from build123d import *

# Parameters (mm, degrees)
BOSS_EXTRUDE1_DEPTH     = 10
CUT_EXTRUDE1_DEPTH      = 333.565782966
CUT_EXTRUDE1_DEPTH_BACK = 333.565782966
SKETCH2_R               = 1.6
FILLET2_R               = 5
CUT_EXTRUDE3_DEPTH      = 333.565782966
CUT_EXTRUDE3_DEPTH_BACK = 333.565782966
SKETCH4_R               = 1.6
FILLET3_R               = 10


with BuildPart() as part:
    # Sketch1 → Boss-Extrude1 (new body)
    with BuildSketch(Plane(origin=(0, 0, 0), x_dir=(1, 0, 0), z_dir=(0, 1, 0))):
        Polygon((0, 120), (0, 151.005050634), (70, 320), (90, 320), (90, 170), (40, 120), (40, 0), (0, 0), align=None)
        Polygon((20, 147.026803286), (70, 267.737481405), (70, 178.284271247), (31.715728753, 140), (20, 140), align=None, mode=Mode.SUBTRACT)
    extrude(amount=BOSS_EXTRUDE1_DEPTH)

    # Sketch2 → Cut-Extrude1 (cut, two sides: drawn at the far end of the back side and taken through both)
    with BuildSketch(Plane(origin=(0, 10, 0), x_dir=(1, 0, 0), z_dir=(0, 1, 0)).offset(-CUT_EXTRUDE1_DEPTH_BACK)):
        with Locations(Location((10, 110, 0), (0, 0, 270))):
            Circle(SKETCH2_R)
        with Locations(Location((30, 110, 0), (0, 0, 270))):
            Circle(SKETCH2_R)
        with Locations(Location((10, 10, 0), (0, 0, 270))):
            Circle(SKETCH2_R)
        with Locations(Location((30, 10, 0), (0, 0, 270))):
            Circle(SKETCH2_R)
    extrude(amount=CUT_EXTRUDE1_DEPTH + CUT_EXTRUDE1_DEPTH_BACK, mode=Mode.SUBTRACT)

    # Fillet2
    fillet2_edges = [part.edges().sort_by_distance(p)[0] for p in [
        (20, 5, -147.026803286),
        (20, 5, -140),
        (31.715728753, 5, -140),
        (70, 5, -178.284271247),
        (70, 5, -267.737481405),
    ]]
    fillet(fillet2_edges, radius=FILLET2_R)

    # Sketch4 → Cut-Extrude3 (cut, two sides: drawn at the far end of the back side and taken through both)
    with BuildSketch(Plane(origin=(0, 10, 0), x_dir=(1, 0, 0), z_dir=(0, 1, 0)).offset(-CUT_EXTRUDE3_DEPTH_BACK)):
        with Locations(Location((85, 310, 0), (0, 0, 270))):
            Circle(SKETCH4_R)
        with Locations(Location((85, 245, 0), (0, 0, 270))):
            Circle(SKETCH4_R)
        with Locations(Location((85, 180, 0), (0, 0, 270))):
            Circle(SKETCH4_R)
    extrude(amount=CUT_EXTRUDE3_DEPTH + CUT_EXTRUDE3_DEPTH_BACK, mode=Mode.SUBTRACT)

    # Fillet3
    fillet3_edges = [part.edges().sort_by_distance(p)[0] for p in [
        (0, 5, -151.005050634),
        (70, 5, -320),
        (90, 5, -320),
        (90, 5, -170),
        (40, 5, -120),
        (40, 5, 0),
        (0, 5, 0),
    ]]
    fillet(fillet3_edges, radius=FILLET3_R)


solid = part.part
CAD build for the part. Positions are in the model's coordinates, mm. A direction names the side the tool comes from. Give positions to 0.01 mm unless a question says otherwise; leave off trailing zeros. Loops run counter-clockwise (first coordinate to the right, second up) from the corner with the lowest first, then second, coordinate; pieces in that order, holes last. Notation, with made-up numbers: M 72.5,59.25 L 119.5,59.25 A21 ccw 119.5,68.25 Z; hole C 78.25,20.5 d5. An arc over 180 degrees is marked long. Write each question's results on one line, items separated by ' | '.
Q1. Band-saw the part on A-A on y = 8. Give the number of separate pieces and of enclosed holes in the cut face, and give its area (3 significant figures).
Geometry check:
separate pieces: 1 | enclosed holes: 8 | area: 13,000 mm²
Q2. Band-saw the part on B-B on x = 52.5. Write the cut outline in (y, z), and give its area (3 significant figures).
Geometry check:
outline: M 0,-277.75 L 10,-277.75 L 10,-225.49 L 0,-225.49 Z; M 0,-160.78 L 10,-160.78 L 10,-132.5 L 0,-132.5 Z | area: 805 mm²
Q3. Probe probe 1 along X at (y, z) = (7.75, -110); probe 2 along Z at (x, y) = (85, 6); probe 3 along X at (y, z) = (4, -180). List the from-to ranges inside material, lowest first.
Geometry check:
probe 1: x = 0 to 8.4, 11.6 to 28.4, 31.6 to 40 | probe 2: z = -318.66 to -311.6, -308.4 to -246.6, -243.4 to -181.6, -178.4 to -165 | probe 3: x = 12.01 to 33.66, 69.99 to 83.4, 86.6 to 90
Q4. Band-saw the part on C-C on z = -156. Write the cut outline in (x, y), and give its area (3 significant figures).
Geometry check:
outline: M 2.07,0 L 23.72,0 L 23.72,10 L 2.07,10 Z; M 47.72,0 L 76,0 L 76,10 L 47.72,10 Z | area: 499 mm²
Q5. Which spindle directions (+Z, -Z, +X, -X, +Y, -Y) get a long thin tool onto all of the face, cutting with end or side? Do faces 5 (the face through (40.1, 4.93, -195.55)), 6 (the face through (90, 5, -243)). Say none if no direction does.
Geometry check:
face 5: +Y, -Y | face 6: +Z, -Z, +X, +Y, -Y
Q6. Band-saw the part on D-D on z = -53.5. Write the cut outline in (x, y).
Geometry check:
outline: M 0,0 L 40,0 L 40,10 L 0,10 Z
Q7. Mould opens along Z. For faces 1 (the face through (65.881, 5.07, -247.523)), 2 (the face through (40, 5, -64)), 3 (the face through (51.105, 4.93, -159.39)), 4 (the face through (2.85, 5.07, -3.01)) say: pulls with the +Z half, pulls with the -Z half, needs draft (parallel to the pull), parting line crosses it, or undercut.
Geometry check:
face 1: undercut | face 2: needs draft | face 3: undercut | face 4: pulls with the +Z half
Q8. Flat gauge pins, fed straight in: P1, Ø3, axis at x = 10, z = -10, coming from the -Y side; P2, Ø3.5, axis at x = 85, z = -310, coming from the +Y side; P3, Ø4, axis at x = 66, y = 3, coming from the +Z side; P4, Ø3, axis at x = 59, y = 4, coming from the -Z side (3 decimals). Where does each tip first touch, or does it go through?
Geometry check:
P1: passes through | P2: stops at y = 10 | P3: stops at z = -144 | P4: stops at z = -297.065
